from build123d import *

# Parameters (mm, degrees)
CROQUIS1_W              = 28
CROQUIS1_H              = 28
CROQUIS1_R              = 8.05
SALIENTE_EXTRUIR1_DEPTH = 0.5
CROQUIS2_W              = 28
CROQUIS2_H              = 28
CROQUIS2_R              = 9.5
SALIENTE_EXTRUIR2_DEPTH = 6.8
CROQUIS7_W              = 2.5
CROQUIS7_H              = 5
CROQUIS7_W_2            = 10
CROQUIS7_H_2            = 4
SALIENTE_EXTRUIR3_DEPTH = 3
REDONDEO1_R             = 5
CROQUIS6_R              = 1.5
CORTAR_EXTRUIR3_DEPTH   = 10


with BuildPart() as part:
    # Croquis1 → Saliente-Extruir1 (new, symmetric)
    with BuildSketch(Plane.XY):
        Rectangle(CROQUIS1_W, CROQUIS1_H)
        Circle(CROQUIS1_R, mode=Mode.SUBTRACT)
    extrude(amount=SALIENTE_EXTRUIR1_DEPTH, both=True)

    # Croquis2 → Saliente-Extruir2 (add)
    with BuildSketch(Plane.XY.offset(0.5)):
        Rectangle(CROQUIS2_W, CROQUIS2_H)
        Circle(CROQUIS2_R, mode=Mode.SUBTRACT)
    extrude(amount=SALIENTE_EXTRUIR2_DEPTH)

    # Croquis7 → Saliente-Extruir3 (add)
    with BuildSketch(Plane(origin=(0, 0, -0.5), x_dir=(-1, 0, 0), z_dir=(0, 0, -1))):
        with Locations((-15.25, 0)):
            Rectangle(CROQUIS7_W, CROQUIS7_H)
        with Locations((0, -16)):
            Rectangle(CROQUIS7_W_2, CROQUIS7_H_2)
        Polygon((14, -2.5), (14, -5), (18.9, -5), (18.9, -2.5), (16.5, -2.5), align=None)
        with Locations((15.25, 0)):
            Rectangle(CROQUIS7_W, CROQUIS7_H)
        Polygon((14, 5), (14, 2.5), (16.5, 2.5), (18.9, 2.5), (18.9, 5), align=None)
    extrude(amount=-SALIENTE_EXTRUIR3_DEPTH)

    # Redondeo1
    redondeo1_edges = [part.edges().sort_by_distance(p)[0] for p in [
        (14, -14, 3.4),
        (-14, -14, 3.4),
        (-14, 14, 3.4),
        (14, 14, 3.4),
    ]]
    fillet(redondeo1_edges, radius=REDONDEO1_R)

    # Croquis6 → Cortar-Extruir3 (cut)
    with BuildSketch(Plane(origin=(0, 0, -0.5), x_dir=(-1, 0, 0), z_dir=(0, 0, -1))):
        with Locations((-9.5, 9.5)):
            Circle(CROQUIS6_R)
        with Locations((9.5, 9.5)):
            Circle(CROQUIS6_R)
        with Locations((9.5, -9.5)):
            Circle(CROQUIS6_R)
        with Locations((-9.5, -9.5)):
            Circle(CROQUIS6_R)
    extrude(amount=-CORTAR_EXTRUIR3_DEPTH, mode=Mode.SUBTRACT)


solid = part.part
The listing builds one solid part. Answer for the finished solid, in the listing's coordinates (mm). A direction names the side the tool comes from. Coordinates: 2 decimals unless noted, no trailing zeros. Loops run counter-clockwise (first coordinate to the right, second up) from the corner with the lowest first, then second, coordinate; pieces in that order, holes last.
1) A tool of negligible diameter and unlimited length cuts with its end or side. For faces 1 (the face through (0, -16, 2.5)), 2 (the face through (-5, -16, 1)), 3 (the face through (5, -16, 1)), 4 (the face through (-18, 2.5, 1)), 5 (the face through (-16, 0, 2.5)), from which of +Z, -Z, +X, -X, +Y, -Y can it reach the whole face along a straight path? Write none if from no direction.
2) Find section D-D on z = 3.5. Write down the section's boundary in (x, y), then the cut area to 3 significant figures.
3) Find section A-A on z = 1. Give the number of separate pieces and of enclosed holes in the cut face, then the cut area to 3 significant figures.
4) Find section C-C on x = 0. Write down the section's boundary in (y, z), then the cut area to 3 significant figures.
5) Find the intervals of material crossed by L1, parallel to Y at x = 0, z = 4.5; L2, parallel to Z at x = 15, y = 0.5; L3, parallel to X at y = 10.5, z = 3.25, in increasing order.
6) Determine the mould class of faces 6 (the face through (10.7, -10.4, 3.3)), 7 (the face through (16.5, 0, 1)), 8 (the face through (12, -13, 3)) for opening direction Y: pulls with the +Y half, pulls with the -Y half, needs draft (parallel to the pull), parting line crosses it, or undercut.
7) Find section B-B on y = 0. Write down the section's boundary in (x, z).
8) Flat-ended cylindrical pins translate along their axes: pin 1 Ø4 at (y, z) = (0.5, 3.5) entering from -X; pin 2 Ø2 at (y, z) = (3.5, 3.5) entering from +X; pin 3 Ø2.5 at (x, z) = (-17.5, 0.5) entering from +Y. Find the tip coordinate at first contact, or state that the pin passes through.
Values:
1. face 1: +Z, +X, -X, -Y
1. face 2: +Z, -Z, -X, -Y
1. face 3: +Z, -Z, +X, -Y
1. face 4: +Z, -Z, -X
1. face 5: +Z, -X, +Y, -Y
2. outline: (-14, -9) arc R5 ccw to (-9, -14) - (9, -14) arc R5 ccw to (14, -9) - (14, 9) arc R5 ccw to (9, 14) - (-9, 14) arc R5 ccw to (-14, 9) - close; hole circle Ø3 at (-9.5, -9.5); hole circle Ø3 at (-9.5, 9.5); hole circle Ø19 at (0, 0); hole circle Ø3 at (9.5, -9.5); hole circle Ø3 at (9.5, 9.5)
2. area: 451 mm2
3. separate pieces: 1
3. enclosed holes: 5
3. area: 540 mm2
4. outline: (-18, -0.5) - (-8.05, -0.5) - (-8.05, 0.5) - (-9.5, 0.5) - (-9.5, 7.3) - (-14, 7.3) - (-14, 2.5) - (-18, 2.5) - close; (8.05, -0.5) - (14, -0.5) - (14, 7.3) - (9.5, 7.3) - (9.5, 0.5) - (8.05, 0.5) - close
4. area: 85.1 mm2
5. L1: y = -14 to -9.5, 9.5 to 14
5. L2: z = -0.5 to 2.5
5. L3: x = -13.77 to -10.62, -8.38 to 8.38, 10.62 to 13.77
6. face 6: undercut
6. face 7: needs draft
6. face 8: pulls with the -Y half
7. outline: (-16.5, -0.5) - (-8.05, -0.5) - (-8.05, 0.5) - (-9.5, 0.5) - (-9.5, 7.3) - (-14, 7.3) - (-14, 2.5) - (-16.5, 2.5) - close; (8.05, -0.5) - (16.5, -0.5) - (16.5, 2.5) - (14, 2.5) - (14, 7.3) - (9.5, 7.3) - (9.5, 0.5) - (8.05, 0.5) - close
8. pin 1: stops at x = -16.5
8. pin 2: stops at x = 14
8. pin 3: stops at y = 5
